from build123d import *

# Parameters (mm, degrees)
AUFSATZ_LINEAR_AUSTRAGEN1_DEPTH = 20
AUFSATZ_LINEAR_AUSTRAGEN2_DEPTH = 15
AUFSATZ_LINEAR_AUSTRAGEN4_DEPTH = 3
SCHNITT_LINEAR_AUSTRAGEN1_REACH = 22
SKIZZE7_W                       = 10
SKIZZE7_H                       = 2
SKIZZE11_W                      = 5
SKIZZE11_H                      = 14.866025404
SCHNITT_LINEAR_AUSTRAGEN4_DEPTH = 10
SKIZZE12_W                      = 5
SKIZZE12_H                      = 19.089107003
AUFSATZ_LINEAR_AUSTRAGEN7_DEPTH = 0.5
SKIZZE13_R                      = 2.5
AUFSATZ_LINEAR_AUSTRAGEN8_DEPTH = 13
SKIZZE8_W                       = 11
SKIZZE8_H                       = 5
SCHNITT_LINEAR_AUSTRAGEN5_DEPTH = 13
FASE1_SIZE                      = 1


with BuildPart() as part:
    # Skizze1 → Aufsatz-Linear austragen1 (new body)
    with BuildSketch(Plane(origin=(0, 0, 0), x_dir=(1, 0, 0), z_dir=(0, 1, 0))):
        Polygon((5.5, -4), (-5.5, -4), (-5.5, -1.5), (-7.5, -1.5), (-7.5, 1.5), (-5.5, 1.5), (-5.5, 4), (5.5, 4), (5.5, 1.5), (7.5, 1.5), (7.5, -1.5), (5.5, -1.5), align=None)
        Polygon((-5, 1), (-5, 3.5), (5, 3.5), (5, 1), (7, 1), (7, -1), (5, -1), (5, -3.5), (-5, -3.5), (-5, -1), (-7, -1), (-7, 1), align=None, mode=Mode.SUBTRACT)
    extrude(amount=AUFSATZ_LINEAR_AUSTRAGEN1_DEPTH)

    # Skizze2 → Aufsatz-Linear austragen2 (add)
    with BuildSketch(Plane.ZY.offset(7.5)):
        Polygon((13.5, 37.320508076), (13.933012702, 37.070508076), (4, 19.866025404), (4, 19.498965661), (1.5, 19.498965661), (1.5, 20), (3.5, 20), align=None)
    extrude(amount=-AUFSATZ_LINEAR_AUSTRAGEN2_DEPTH)

    # Skizze6 → Aufsatz-Linear austragen4 (add)
    with BuildSketch(Plane.ZY.offset(5.5)):
        Polygon((13.933012702, 37.070508076), (4, 0), (4, 19.866025404), align=None)
    aufsatz_linear_austragen4 = extrude(amount=-AUFSATZ_LINEAR_AUSTRAGEN4_DEPTH)

    # Skizze7 → Schnitt-Linear austragen1 (cut, up to next)
    with BuildSketch(Plane(origin=(0, 20, 0), x_dir=(1, 0, 0), z_dir=(0, 1, 0)), mode=Mode.PRIVATE) as schnitt_linear_austragen1_sk1:
        with Locations((0, -2.5)):
            Rectangle(SKIZZE7_W, SKIZZE7_H)
    schnitt_linear_austragen1_tool1 = extrude(schnitt_linear_austragen1_sk1.sketch, amount=-SCHNITT_LINEAR_AUSTRAGEN1_REACH, mode=Mode.PRIVATE) & part.part
    add(schnitt_linear_austragen1_tool1.solids().sort_by_distance((0, 20, 2.5))[0], mode=Mode.SUBTRACT)

    # Spiegeln3: Aufsatz-Linear austragen4 across plane
    add(aufsatz_linear_austragen4.mirror(Plane(origin=(0, 0, 0), x_dir=(0, 0, 1), z_dir=(1, 0, 0))))

    # Skizze11 → Schnitt-Linear austragen4 (cut)
    with BuildSketch(Plane(origin=(0, 3.234455543, -5.602241336), x_dir=(1, 0, 0), z_dir=(0, -0.5, 0.866025404))):
        with Locations((0, 26.637495374)):
            Rectangle(SKIZZE11_W, SKIZZE11_H)
    extrude(amount=-SCHNITT_LINEAR_AUSTRAGEN4_DEPTH, mode=Mode.SUBTRACT)

    # Skizze12 → Aufsatz-Linear austragen7 (add)
    with BuildSketch(Plane(origin=(0, -1, 3.732050808), x_dir=(1, 0, 0), z_dir=(0, -0.258819045, 0.965925826))):
        with Locations((-5, 29.768936686)):
            Rectangle(SKIZZE12_W, SKIZZE12_H)
    aufsatz_linear_austragen7 = extrude(amount=AUFSATZ_LINEAR_AUSTRAGEN7_DEPTH)

    # Spiegeln4: Aufsatz-Linear austragen7 across plane
    add(aufsatz_linear_austragen7.mirror(Plane(origin=(0, 0, 0), x_dir=(0, 0, 1), z_dir=(1, 0, 0))))

    # Skizze13 → Aufsatz-Linear austragen8 (add)
    with BuildSketch(Plane(origin=(5.5, 0, 0), x_dir=(0, 0, -1), z_dir=(1, 0, 0))):
        with Locations((-8.069309397, 22.914276031)):
            Circle(SKIZZE13_R)
    aufsatz_linear_austragen8 = extrude(amount=AUFSATZ_LINEAR_AUSTRAGEN8_DEPTH)

    # Skizze8 → Schnitt-Linear austragen5 (cut)
    with BuildSketch(Plane(origin=(0, 0, 3.5), x_dir=(-1, 0, 0), z_dir=(0, 0, -1))):
        with Locations((0, 2.5)):
            Rectangle(SKIZZE8_W, SKIZZE8_H)
    extrude(amount=-SCHNITT_LINEAR_AUSTRAGEN5_DEPTH, mode=Mode.SUBTRACT)

    # Spiegeln5: Aufsatz-Linear austragen8 across plane
    add(aufsatz_linear_austragen8.mirror(Plane(origin=(0, 0, 0), x_dir=(0, 0, 1), z_dir=(1, 0, 0))))

    # Fase1
    fase1_edges = [part.edges().sort_by_distance(p)[0] for p in [
        (-7.5, 18.470549277, 9.207987808),
        (7.5, 18.470549277, 9.207987808),
        (18.5, 22.914276031, 10.569309397),
        (-18.5, 22.914276031, 10.569309397),
    ]]
    chamfer(fase1_edges, length=FASE1_SIZE)


solid = part.part
Read the model definition and answer for the solid it produces. Units are mm, in the model's axes. A direction names the side the tool comes from. Give positions to 0.01 mm unless a question says otherwise; leave off trailing zeros. Loops run counter-clockwise (first coordinate to the right, second up) from the corner with the lowest first, then second, coordinate; pieces in that order, holes last. Notation, with made-up numbers: (2, -16) - (35, -16) arc R15 ccw to (35, 2) - close; hole circle Ø5 at (50, -28.75). An arc over 180 degrees is marked (long way). Answer as CSV lines item,"result". Start each with the question number.
1) Which of the six approach directions +Z, -Z, +X, -X, +Y, -Y give full straight-line access (tool end or side, diameter ignored) to faces 5 (the face through (7, 10, 0)), 6 (the face through (5.5, 29, 10)), 7 (the face through (5.5, 10, -3)), 8 (the face through (0, 10, -4))?
2) Find section C-C (y = 28). Write down the section's boundary in (x, z).
3) Determine the mould class of faces 1 (the face through (6.486, 31.225, 10.558)), 2 (the face through (2.5, 21, 8)), 3 (the face through (-7.5, 20.5, 9.8)), 4 (the face through (7.5, 30.77, 9.94)) for opening direction X: released by +X, released by -X, zero draft, split by the parting line, or undercut.
4) Each of these flat-tipped pins is pushed along its axis until it touches: pin 1 Ø2 at (y, z) = (8, 2) entering from -X; pin 2 Ø1.6 at (x, z) = (-7, 3) entering from -Y; pin 3 Ø2 at (x, z) = (6, 11) entering from +Y; pin 4 Ø1 at (x, z) = (10.5, 12) entering from +Y. Where does it stop, or does it pass through?
5) Find section B-B (x = -3). Write down the section's boundary in (y, z).
6) Find section D-D (y = 4.5). Write down the section's boundary in (x, z).
7) Straight lines are drawn through the part: L1, parallel to X at y = 14.5, z = -0.5; L2, parallel to X at y = 28, z = 10.5; L3, parallel to Z at x = 1.5, y = 13. For each, find the intervals that lie inside material, in ascending order. Write a range as from..to.
8) Find section A-A (z = 2.5). Write down the section's boundary in (x, y), then the cut area to 3 significant figures.
Findings below:
1,face 5,"+Y, -Y"
1,face 6,"+X"
1,face 7,"-Z, +X, +Y, -Y"
1,face 8,"-Z, +X, -X, +Y, -Y"
2,outline,"(-7.5, 8.12) - (-2.5, 8.12) - (-2.5, 12.02) - (-7.5, 12.02) - (-7.5, 11.5) - (-5.5, 11.5) - (-5.5, 8.7) - (-7.5, 8.7) - close; (2.5, 8.12) - (7.5, 8.12) - (7.5, 8.7) - (5.5, 8.7) - (5.5, 11.5) - (7.5, 11.5) - (7.5, 12.02) - (2.5, 12.02) - close"
3,face 1,"zero draft"
3,face 2,"undercut"
3,face 3,"released by -X"
3,face 4,"released by +X"
4,pin 1,"x = -7.5"
4,pin 2,"y = 19.5"
4,pin 3,"y = 34.72"
4,pin 4,"through"
5,outline,"(0, -4) - (20, -4) - (20, -3.5) - (0, -3.5) - close; (5, 3.5) - (20, 3.5) - (37.32, 13.5) - (37.07, 13.93) - (36.97, 13.91) - (36.84, 14.39) - (18.41, 9.45) - (18.54, 8.97) - (5, 5.34) - close"
6,outline,"(-7.5, -1.5) - (-5.5, -1.5) - (-5.5, -4) - (5.5, -4) - (5.5, -1.5) - (7.5, -1.5) - (7.5, 1.5) - (5.5, 1.5) - (5.5, 3.5) - (5, 3.5) - (5, 1) - (7, 1) - (7, -1) - (5, -1) - (5, -3.5) - (-5, -3.5) - (-5, -1) - (-7, -1) - (-7, 1) - (-5, 1) - (-5, 3.5) - (-5.5, 3.5) - (-5.5, 1.5) - (-7.5, 1.5) - close"
7,L1,"-7.5..-7, 7..7.5"
7,L2,"-5.5..-2.5, 2.5..5.5"
7,L3,"-4..-3.5, 3.5..4"
8,outline,"(-7.5, 19.5) - (-5.5, 19.5) - (-5.5, 0) - (-5, 0) - (-5, 20) - (-7.5, 20) - close; (5, 0) - (5.5, 0) - (5.5, 19.5) - (7.5, 19.5) - (7.5, 20) - (5, 20) - close"
8,area,"22.0 mm^2"
